from build123d import *

# Parameters (mm, degrees)
BOSS_SWITCHMAIN_DEPTH           = 3
SKETCH1_W                       = 6.582729781
SKETCH1_H                       = 1.5
SKETCH1_W_2                     = 3.025930853
SKETCH1_W_3                     = 4.49100728
BOSS_FLANGE_WIDTH_DEPTH         = 6
SKETCH2_W                       = 5
SKETCH2_H                       = 1.5
BOSS_FLANGE_HEIGHT_DEPTH        = 11.6675
TAP_DRILL_FOR_M2X0_4_TAP1_D     = 1.6
M2_CLEARANCE_HOLE2_D            = 2.4
M2_CLEARANCE_HOLE2_DEPTH        = 6.113984988
M2_CLEARANCE_HOLE2_TIP          = 0.721032743
CUT_FLANGE_RAMP_CLEARANCE_REACH = 19.959
SKETCH10_W                      = 1.51157113
SKETCH10_H                      = 3
CUT_EXTRUDE1_REACH              = 28.283
CUT_EXTRUDE2_REACH              = 22.07


with BuildPart() as part:
    # Sketch-SwitchBossUp → Boss-SwitchMain (new body)
    with BuildSketch(Plane.XY):
        with BuildLine():
            Line((6.540476927, 22.165014537), (6.540476927, 25.093856925))
            Line((6.540476927, 25.093856925), (8.540476927, 25.093856925))
            Line((8.540476927, 25.093856925), (8.540476927, 20.473554675))
            Line((8.540476927, 20.473554675), (2.463355023, 19.450530066))
            Line((2.463355023, 19.450530066), (3.113617204, 15.587746603))
            ThreePointArc((3.113617204, 15.587746603), (2.228151344, 14.454516392), (3.25659329, 13.449246446))
            ThreePointArc((3.25659329, 13.449246446), (4.285298124, 14.079636296), (4.085366752, 15.269448233))
            Line((4.085366752, 15.269448233), (3.613617204, 15.269448233))
            Line((3.613617204, 15.269448233), (3.613617204, 16.769448233))
            Line((3.613617204, 16.769448233), (6.639548057, 16.769448233))
            Line((6.639548057, 16.769448233), (6.639548057, 14.40837951))
            Line((6.639548057, 14.40837951), (5.90556854, 14.440674771))
            ThreePointArc((5.90556854, 14.440674771), (4.876863705, 13.810284921), (5.076795077, 12.620472983))
            Line((5.076795077, 12.620472983), (4.742765687, 11.886857682))
            ThreePointArc((4.742765687, 11.886857682), (4.116092357, 11.977881728), (3.546393548, 11.701389219))
            ThreePointArc((3.546393548, 11.701389219), (3.274676841, 10.525891439), (4.263259905, 9.834278449))
            ThreePointArc((4.263259905, 9.834278449), (4.46894162, 9.850585257), (4.667751547, 9.905771245))
            Line((4.667751547, 9.905771245), (6.093996382, 10.453369682))
            Line((6.093996382, 10.453369682), (6.73413388, 9.742424966))
            Line((6.73413388, 9.742424966), (6.73413388, 8.198043394))
            Line((6.73413388, 8.198043394), (6.493366278, 8.105602069))
            Line((6.493366278, 8.105602069), (5.504663813, 7.725995489))
            ThreePointArc((5.504663813, 7.725995489), (5.320005472, 7.633951058), (5.156260325, 7.508418563))
            ThreePointArc((5.156260325, 7.508418563), (4.884543619, 6.332920783), (5.873126682, 5.641307794))
            ThreePointArc((5.873126682, 5.641307794), (6.898907846, 4.833576465), (6.394232666, 3.629433676))
            Line((6.394232666, 3.629433676), (5.040476927, 2.847842436))
            Line((5.040476927, 2.847842436), (5.040476927, -1.189543551))
            Line((5.040476927, -1.189543551), (-1.954752854, -1.189543551))
            Line((-1.954752854, -1.189543551), (-1.954752854, 4.924441437))
            Line((-1.954752854, 4.924441437), (2.536254426, 4.924441437))
            ThreePointArc((2.536254426, 4.924441437), (3.271135169, 4.635221221), (4.006015912, 4.924441437))
            ThreePointArc((4.006015912, 4.924441437), (4.277732619, 6.099939217), (3.289149555, 6.791552207))
            Line((3.289149555, 6.791552207), (2.396149135, 9.117412093))
            ThreePointArc((2.396149135, 9.117412093), (2.667865841, 10.292909873), (1.679282778, 10.984522862))
            ThreePointArc((1.679282778, 10.984522862), (0.990609652, 11.24824473), (0.632497087, 11.892896022))
            Line((0.632497087, 11.892896022), (-0.448028681, 18.3115948))
            ThreePointArc((-0.448028681, 18.3115948), (-0.266285833, 19.102309392), (0.421345416, 19.532917442))
            Line((0.421345416, 19.532917442), (-0.465233701, 24.799505683))
            ThreePointArc((-0.465233701, 24.799505683), (-2.406587703, 25.978955839), (-3.001107523, 28.171329943))
            ThreePointArc((-3.001107523, 28.171329943), (-2.220760115, 28.789797628), (-1.602292431, 28.009450221))
            ThreePointArc((-1.602292431, 28.009450221), (0.141134159, 26.168671513), (1.647974165, 28.207650602))
            ThreePointArc((1.647974165, 28.207650602), (2.167041147, 29.057364566), (3.016755111, 28.538297585))
            ThreePointArc((3.016755111, 28.538297585), (2.839798095, 26.578800421), (1.507016259, 25.131514861))
            Line((1.507016259, 25.131514861), (2.131345845, 21.422780026))
            Line((2.131345845, 21.422780026), (6.540476927, 22.165014537))
        make_face()
    extrude(amount=BOSS_SWITCHMAIN_DEPTH)

    # Sketch1 → Boss-Flange Width (add)
    with BuildSketch(Plane(origin=(0, 0, 0), x_dir=(-1, 0, 0), z_dir=(0, 0, -1))):
        with Locations((-1.336612037, -0.439543551)):
            Rectangle(SKETCH1_W, SKETCH1_H)
        with Locations((-5.126582631, 16.019448233)):
            Rectangle(SKETCH1_W_2, SKETCH1_H)
        with Locations((-0.290750786, 4.174441437)):
            Rectangle(SKETCH1_W_3, SKETCH1_H)
    extrude(amount=BOSS_FLANGE_WIDTH_DEPTH)

    # Sketch2 → Boss-Flange Height (add)
    with BuildSketch(Plane(origin=(-7.039523073, 0, 0), x_dir=(0, 0, -1), z_dir=(1, 0, 0))):
        with Locations((3.5, 16.019448233)):
            Rectangle(SKETCH2_W, SKETCH2_H)
        with Locations((3.5, 4.174441437)):
            Rectangle(SKETCH2_W, SKETCH2_H)
        with Locations((3.5, -0.439543551)):
            Rectangle(SKETCH2_W, SKETCH2_H)
    extrude(amount=BOSS_FLANGE_HEIGHT_DEPTH)

    # Tap Drill for M2x0.4 Tap1 (through all)
    with Locations(Plane(origin=(0, -1.189543551, 0), x_dir=(-1, 0, 0), z_dir=(0, -1, 0))):
        with Locations((4.039523073, 3.5), (-1.627976927, 3.5)):
            Hole(TAP_DRILL_FOR_M2X0_4_TAP1_D / 2)

    # M2 Clearance Hole2
    with Locations(Plane.XZ.offset(1.189543551)):
        with Locations((-4.039523073, -3.5), (1.627976927, -3.5)):
            Hole(M2_CLEARANCE_HOLE2_D / 2, depth=M2_CLEARANCE_HOLE2_DEPTH)
            with Locations((0, 0, -(M2_CLEARANCE_HOLE2_DEPTH + M2_CLEARANCE_HOLE2_TIP / 2))):  # 118° drill point
                Cone(0, M2_CLEARANCE_HOLE2_D / 2, M2_CLEARANCE_HOLE2_TIP, mode=Mode.SUBTRACT)

    # Sketch10 → Cut-Flange Ramp Clearance (cut, up to next)
    with BuildSketch(Plane(origin=(0, 16.769448233, 0), x_dir=(1, 0, 0), z_dir=(0, 1, 0)), mode=Mode.PRIVATE) as cut_flange_ramp_clearance_sk1:
        with Locations((5.883762492, 4.5)):
            Rectangle(SKETCH10_W, SKETCH10_H)
    cut_flange_ramp_clearance_tool1 = extrude(cut_flange_ramp_clearance_sk1.sketch, amount=-CUT_FLANGE_RAMP_CLEARANCE_REACH, mode=Mode.PRIVATE) & part.part
    add(cut_flange_ramp_clearance_tool1.solids().sort_by_distance((5.883762, 16.769448, -4.5))[0], mode=Mode.SUBTRACT)

    # Sketch12 → Cut-Extrude1 (cut, up to next)
    with BuildSketch(Plane(origin=(0, 25.093856925, 0), x_dir=(1, 0, 0), z_dir=(0, 1, 0)), mode=Mode.PRIVATE) as cut_extrude1_sk1:
        Polygon((6.540476927, 0), (8.540476927, -3), (8.540476927, 0), align=None)
    cut_extrude1_tool1 = extrude(cut_extrude1_sk1.sketch, amount=-CUT_EXTRUDE1_REACH, mode=Mode.PRIVATE) & part.part
    add(cut_extrude1_tool1.solids().sort_by_distance((7.87381, 25.093857, 1))[0], mode=Mode.SUBTRACT)

    # Sketch14 → Cut-Extrude2 (cut, up to next)
    with BuildSketch(Plane(origin=(3.789105765, 8.959047136, -3.436717579), x_dir=(-0.930109907, 0.342916579, -0.131543837), z_dir=(-0.367281311, -0.868408215, 0.333124018)), mode=Mode.PRIVATE) as cut_extrude2_sk1:
        Polygon((-0.94466877, -3.547806869), (-4.277307049, -3.078270724), (-4.824829049, -6.964431121), (-1.431952972, -6.964431121), align=None)
    cut_extrude2_tool1 = extrude(cut_extrude2_sk1.sketch, amount=-CUT_EXTRUDE2_REACH, mode=Mode.PRIVATE) & part.part
    add(cut_extrude2_tool1.solids().sort_by_distance((6.491643, 9.802029, 1.740466))[0], mode=Mode.SUBTRACT)


solid = part.part
Input: part model. Units: mm. Frame: model coordinates. A direction names the side the tool comes from. Coordinates: 2 decimals unless noted, no trailing zeros. Loops run counter-clockwise (first coordinate to the right, second up) from the corner with the lowest first, then second, coordinate; pieces in that order, holes last.
Q1. Cut plane D-D (y = 17.5). Output: boundary loops of the cut face in (x, z).
Q2. Cut plane B-B (x = 0). Output: boundary loops of the cut face in (y, z).
Q3. Contact query for flat-ended pins moving along their axis: pin 1 (1.8 mm diameter, centred on x = -4.04, z = -3.5, fed in from -Y); pin 2 (1.6 mm diameter, centred on y = 0, z = -4, fed in from +X); pin 3 (1 mm diameter, centred on x = 7, z = 2, fed in from +Y). Output: stop coordinate, or through.
Q4. Material intervals for line 1 (Y direction, x = 0.25, z = -4); line 2 (X direction, y = 15.7, z = -3.5); line 3 (Y direction, x = -0.25, z = -0.75), sorted ascending.
Q5. Cut plane A-A (y = 4). Output: boundary loops of the cut face in (x, z).
Q6. Set-up query: faces 1 (the face through (2.85, 7.94, 1.48)), 2 (the face through (5.128, 16, -4)), 3 (the face through (-5, 0, -1)), 4 (the face through (0.1, 15.06, 1.48)), 5 (the face through (3.614, 16, 1)). Return all of +Z, -Z, +X, -X, +Y, -Y with unobstructed straight access to the full face (end or side cutting, diameter ignored); none if empty.
Q7. Draft query along Y for faces 6 (the face through (7.526, 22.65, 1.479)), 7 (the face through (5.945, 9.776, 1.069)), 8 (the face through (7, 25.094, 2)), 9 (the face through (5.054, 10.054, 2.146)). Return one class per face: +Y half, -Y half, draft (parallel to the pull), parting line (faces both ways), or undercut.
Q8. Cut plane C-C (z = -3.5). Give the number of separate pieces and of enclosed holes in the cut face, then the cut area to 3 significant figures.
Working result:
1. outline: (-0.31, 0) - (2.79, 0) - (2.79, 3) - (-0.31, 3) - close
2. outline: (-1.19, -6) - (0.31, -6) - (0.31, 0) - (3.42, 0) - (3.42, -6) - (4.92, -6) - (4.92, 3) - (-1.19, 3) - close; (15.27, -6) - (16.77, -6) - (16.77, -1) - (15.27, -1) - close; (15.65, 0) - (19.36, 0) - (19.36, 3) - (15.65, 3) - close; (22.04, 0) - (26.17, 0) - (26.17, 3) - (22.04, 3) - close
3. pin 1: stops at y = 15.27
3. pin 2: stops at x = 4.63
3. pin 3: stops at y = 25.09
4. line 1: y = -1.19 to 0.31, 3.42 to 4.92, 15.27 to 16.77
4. line 2: x = -7.04 to -4.84, -3.24 to 0.83, 2.43 to 5.13
4. line 3: y = -1.19 to 0.31, 3.42 to 4.92
5. outline: (-7.04, -6) - (4.63, -6) - (4.63, -1) - (2.54, -1) - (2.54, 0) - (6.77, 0) - (6.77, 3) - (-1.95, 3) - (-1.95, -1) - (-7.04, -1) - close; hole circle Ø2.4 at (-4.04, -3.5); hole circle Ø2.4 at (1.63, -3.5)
6. face 1: +Z, -Z, -X
6. face 2: -Z, +X, +Y, -Y
6. face 3: +Z, -X, +Y, -Y
6. face 4: +Z, -X
6. face 5: +Z
7. face 6: draft
7. face 7: undercut
7. face 8: +Y half
7. face 9: undercut
8. separate pieces: 9
8. enclosed holes: 0
8. area: 34.1 mm2
